from build123d import *

# Parameters (mm, degrees)
SKETCH_1_W          = 18
SKETCH_1_H          = 18
EXTRUDE_1_DEPTH     = 8
CUT_EXTRUDE_START   = 8
SKETCH_5_W          = 16
SKETCH_5_H          = 17
CUT_EXTRUDE_6_DEPTH = 7
EXTRUDE_START       = 8
SKETCH_6_W          = 18
SKETCH_6_H          = 18
EXTRUDE_2_DEPTH     = 1
CUT_EXTRUDE_START_2 = 9
SKETCH_7_R          = 6.5
CUT_EXTRUDE_7_DEPTH = 1
SKETCH_10_W         = 18
SKETCH_10_H         = 18
CUT_EXTRUDE_8_DEPTH = 1


with BuildPart() as part:
    # 스케치1 → 보스-돌출1 (new body)
    with BuildSketch(Plane(origin=(0, 0, 0), x_dir=(1, 0, 0), z_dir=(0, 1, 0))):
        Rectangle(SKETCH_1_W, SKETCH_1_H)
    extrude(amount=EXTRUDE_1_DEPTH)

    # 스케치5 → 컷-돌출6 (cut)
    with BuildSketch(Plane(origin=(0, 0, 0), x_dir=(1, 0, 0), z_dir=(0, 1, 0)).offset(CUT_EXTRUDE_START)):
        with Locations((0, 0.5)):
            Rectangle(SKETCH_5_W, SKETCH_5_H)
    extrude(amount=-CUT_EXTRUDE_6_DEPTH, mode=Mode.SUBTRACT)


with BuildPart() as body_2:
    # 스케치6 → 보스-돌출2 (new body)
    with BuildSketch(Plane(origin=(0, 0, 0), x_dir=(1, 0, 0), z_dir=(0, 1, 0)).offset(EXTRUDE_START)):
        Rectangle(SKETCH_6_W, SKETCH_6_H)
    extrude(amount=EXTRUDE_2_DEPTH)

    # 스케치7 → 컷-돌출7 (cut)
    with BuildSketch(Plane(origin=(0, 0, 0), x_dir=(1, 0, 0), z_dir=(0, 1, 0)).offset(CUT_EXTRUDE_START_2)):
        with Locations(Location((0, -0.5, 0), (0, 0, 270))):
            Circle(SKETCH_7_R)
    extrude(amount=-CUT_EXTRUDE_7_DEPTH, mode=Mode.SUBTRACT)

    # 스케치10 → 컷-돌출8 (cut)
    with BuildSketch(Plane(origin=(0, 9, 0), x_dir=(1, 0, 0), z_dir=(0, 1, 0))):
        Rectangle(SKETCH_10_W, SKETCH_10_H)
    extrude(amount=-CUT_EXTRUDE_8_DEPTH, mode=Mode.SUBTRACT)


solid = part.part
The model under review builds one solid part; all positions refer to its coordinate system, in mm. A direction names the side the tool comes from. Round coordinates to 2 decimals unless told otherwise and drop trailing zeros. Order: outer loops, then holes, each group sorted by start corner. A loop starts at its lowest first (then second) coordinate and runs counter-clockwise, first axis right, second up. Notation, with made-up numbers: (22.5, -25.5) -> (60.5, -25.5) arc R29 ccw to (60.5, 9.5) -> close; hole circle Ø7 at (29.25, 67.25). An arc over 180 degrees is marked (long way). Write item = value, one per line. Start each with the question number.
Item 1: Consider section B-B on z = 7.5. Write out the cut boundary in (x, y).
Item 2: For faces 1 (the face through (0, 0, 0)), 2 (the face through (0, 5, 8)), list the 3-axis set-ups (+Z, -Z, +X, -X, +Y, -Y) from which the entire face can be reached by the end or side of a thin tool; tool diameter is ignored.
Item 3: Clearance check with a flat-ended pin moving along its axis: pin 1 Ø3 at (x, y) = (-3, 6) entering from -Z. State where the tip first meets the part, or that it passes through.
Item 4: Consider section C-C on x = 4. Write out the cut boundary in (y, z), plus the area to 3 significant figures.
Item 5: Consider section A-A on y = 1.5. Write out the cut boundary in (x, z).
Item 6: For line 1 along X through (y, z) = (3.75, -5.5); line 2 along Y through (x, z) = (-0.5, -0.25); line 3 along Z through (x, y) = (1, 1.5), list the stretches that pass through material, from the lowest coordinate up.
Conclusion:
q1.outline = (-9, 0) -> (9, 0) -> (9, 8) -> (8, 8) -> (8, 1) -> (-8, 1) -> (-8, 8) -> (-9, 8) -> close
q2.face_1 = +Z, -Z, +X, -X, -Y
q2.face_2 = -Z, +Y
q3.pin_1 = 8
q4.outline = (0, -9) -> (1, -9) -> (1, 8) -> (8, 8) -> (8, 9) -> (0, 9) -> close
q4.area = 25.0 mm2
q5.outline = (-9, -9) -> (-8, -9) -> (-8, 8) -> (8, 8) -> (8, -9) -> (9, -9) -> (9, 9) -> (-9, 9) -> close
q6.line_1 = -9 to -8, 8 to 9
q6.line_2 = 0 to 1
q6.line_3 = 8 to 9
